The listing builds one solid part. Answer for the finished solid, in the listing's coordinates (mm). Face numbers are marked on the shaded views. Give positions to 0.01 mm unless a question says otherwise; leave off trailing zeros. Write each loop counter-clockwise with the first axis right and the second up, starting at its lowest first coordinate (ties: lowest second). Pieces come first, ordered by that corner, then holes. Notation, with made-up numbers: (67.25, -4.5) - (124.25, -4.5) arc R28 cw to (124.25, 16.5) - close; hole circle Ø4 at (67.25, -18). An arc over 180 degrees is marked (long way). Write each question's results on one line, items separated by ' | '. Start each with the question number.
Q1. Flat-ended cylindrical pins translate along their axes: pin 1 Ø6 at (x, z) = (-24.5, 12.5) entering from -Y; pin 2 Ø3 at (x, z) = (-7.5, -24) entering from -Y; pin 3 Ø4 at (x, z) = (-24.5, 21.5) entering from -Y. Find the tip coordinate at first contact, or state that the pin passes through.
Q2. Section A-A (z = 0) is taken. Determine the outline of the cut face in (x, y), plus the area to 3 significant figures.
Q3. For a pull along Z with two mould halves and no side action, classify the marked faces 1, 2 and 3 as pulls with the +Z half, pulls with the -Z half, needs draft (parallel to the pull), parting line crosses it, or undercut.
Q4. Find the intervals of material crossed by probe 1 along Y at (x, z) = (-24.5, 11); probe 2 along Y at (x, z) = (-16.5, -4); probe 3 along X at (y, z) = (41, -3.5), in increasing order.
Q5. Section B-B (x = -16) is taken. Determine the outline of the cut face in (y, z), plus the area to 3 significant figures.
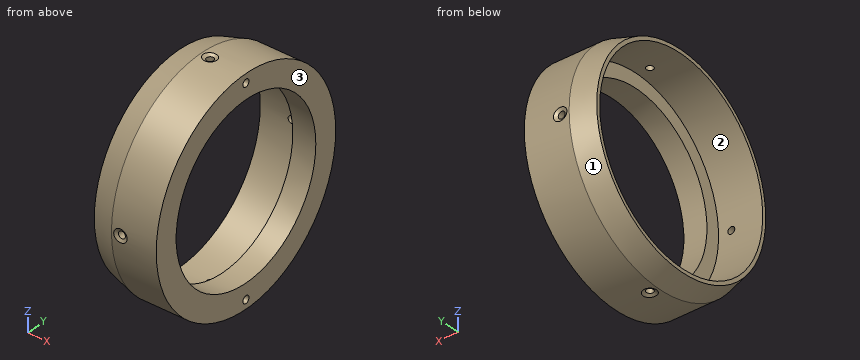
```python
from build123d import *

# Parameters (mm, degrees)
CHANFREIN1_SIZE              = 10
CHANFREIN1_SIZE2             = 2.867453858
R_P_TITION_CIRCULAIRE1_COUNT = 2
R_P_TITION_CIRCULAIRE2_COUNT = 4


with BuildPart() as part:
    # Esquisse1 → Révolution1 (revolve)
    with BuildSketch(Plane.XY):
        Polygon((0, 49), (0, 38.15), (-10.3, 38.15), (-10.3, 44.5), (-30, 44.5), (-30, 49), align=None)
    revolve(axis=Axis((-37.547636856, 0, 0), (1, 0, 0)))

    # Chanfrein1
    chanfrein1_edges = [part.edges().sort_by_distance(p)[0] for p in [
        (-30, -49, 0),
    ]]
    chanfrein1_side = [part.faces().sort_by_distance(p)[0] for p in [
        (-15, -49, 0),
    ]]
    chamfer(chanfrein1_edges, length=CHANFREIN1_SIZE, length2=CHANFREIN1_SIZE2, reference=chanfrein1_side[0])

    # Esquisse6 → Trou taraudé M41 (revolve, cut)
    with BuildSketch(Plane(origin=(0, 0, -45), x_dir=(0, 0, -1), z_dir=(0, 1, 0))):
        Polygon((0, 0), (0, 7.991420021), (1.65, 7), (1.65, 0), align=None)
    trou_taraud_m41 = revolve(axis=Axis((6.35, 0, -45), (-1, 0, 0)), mode=Mode.SUBTRACT)

    # Répétition circulaire1: Trou taraudé M41 ×2 about axis
    r_p_tition_circulaire1_axis = Axis((0, 0, 0), (1, 0, 0))
    for i in range(1, R_P_TITION_CIRCULAIRE1_COUNT):
        add(trou_taraud_m41.rotate(r_p_tition_circulaire1_axis, i * 360 / R_P_TITION_CIRCULAIRE1_COUNT), mode=Mode.SUBTRACT)

    # Esquisse8 → Dégagement M2.51 (revolve, cut)
    with BuildSketch(Plane(origin=(-16, 0, -49), x_dir=(0, 1, 0), z_dir=(1, 0, 0))):
        Polygon((0, 0), (0, 20.931333959), (1.55, 20), (1.55, 0.83715789), (3, 0), align=None)
    d_gagement_m2_51 = revolve(axis=Axis((-16, 0, -55.35), (0, 0, 1)), mode=Mode.SUBTRACT)

    # Répétition circulaire2: Dégagement M2.51 ×4 about axis
    r_p_tition_circulaire2_axis = Axis((0, 0, 0), (-1, 0, 0))
    for i in range(1, R_P_TITION_CIRCULAIRE2_COUNT):
        add(d_gagement_m2_51.rotate(r_p_tition_circulaire2_axis, i * 360 / R_P_TITION_CIRCULAIRE2_COUNT), mode=Mode.SUBTRACT)


solid = part.part
```
Answers below:
1) pin 1: stops at y = -47.2 | pin 2: stops at y = -43.53 | pin 3: stops at y = -43.74
2) outline: (-30, -46.13) - (-20, -49) - (-19, -49) - (-17.55, -48.16) - (-17.55, -44.5) - (-30, -44.5) - close; (-30, 44.5) - (-17.55, 44.5) - (-17.55, 48.16) - (-19, 49) - (-20, 49) - (-30, 46.13) - close; (-14.45, -48.16) - (-13, -49) - (0, -49) - (0, -38.15) - (-10.3, -38.15) - (-10.3, -44.5) - (-14.45, -44.5) - close; (-14.45, 44.5) - (-10.3, 44.5) - (-10.3, 38.15) - (0, 38.15) - (0, 49) - (-13, 49) - (-14.45, 48.16) - close | area: 342 mm2
3) face 1: parting line crosses it | face 2: undercut | face 3: needs draft
4) probe 1: y = -46.42 to -43.12, 43.12 to 46.42 | probe 2: y = -48.84 to -44.32, 44.32 to 48.84 | probe 3: x = -10.3 to 0
5) outline: (-48.92, -2.86) arc R49 ccw to (-2.86, -48.92) - (-1.55, -48.16) - (-1.55, -44.47) arc R44.5 cw to (-44.47, -1.55) - (-48.16, -1.55) - close; (-48.92, 2.86) - (-48.16, 1.55) - (-44.47, 1.55) arc R44.5 cw to (-1.55, 44.47) - (-1.55, 48.16) - (-2.86, 48.92) arc R49 ccw to start; (1.55, -48.16) - (2.86, -48.92) arc R49 ccw to (48.92, -2.86) - (48.16, -1.55) - (44.47, -1.55) arc R44.5 cw to (1.55, -44.47) - close; (1.55, 44.47) arc R44.5 cw to (44.47, 1.55) - (48.16, 1.55) - (48.92, 2.86) arc R49 ccw to (2.86, 48.92) - (1.55, 48.16) - close | area: 1,260 mm2
